Can you work these out from the model? Positions are in its coordinate system, mm. A direction names the side the tool comes from. Round coordinates to 2 decimals unless told otherwise and drop trailing zeros. Loops run counter-clockwise (first coordinate to the right, second up) from the corner with the lowest first, then second, coordinate; pieces in that order, holes last. Notation, with made-up numbers: (74, -9) -> (114, -9) arc R8 cw to (114, 2) -> close; hole circle Ø9 at (84, -33.5). An arc over 180 degrees is marked (long way). Answer as a JSON object with one key per item and string values.
```python
from build123d import *

# Parameters (mm, degrees)
EXTRUDE_THIN4_DEPTH   = 96.52
EXTRUDE_THIN4_2_DEPTH = 96.52
SKETCH5_W             = 32.004
SKETCH5_H             = 76.792210726
CUT_EXTRUDE2_DEPTH    = 26.67
SKETCH6_W             = 32.512
SKETCH6_H             = 76.792210726
CUT_EXTRUDE3_DEPTH    = 26.67
SKETCH7_W             = 152.4
SKETCH7_H             = 25.4
BOSS_EXTRUDE1_DEPTH   = 26.67
BOSS_EXTRUDE2_DEPTH   = 12.7
SKETCH13_W            = 25.4
SKETCH13_H            = 19.05
BOSS_EXTRUDE3_DEPTH   = 12.7


with BuildPart() as part:
    # Sketch1 → Extrude-Thin4 (new body)
    with BuildSketch(Plane(origin=(0, 0, 0), x_dir=(0, 0, -1), z_dir=(1, 0, 0))):
        Polygon((19.05, -1.27), (55.88, -1.27), (55.88, -50.207789274), (-2.03892683, -98.807539415), (-0.406246301, -100.753292301), (58.42, -51.392210726), (58.42, 1.27), (19.05, 1.27), align=None)
    extrude(amount=EXTRUDE_THIN4_DEPTH)

    # Sketch6 → Cut-Extrude3 (cut)
    with BuildSketch(Plane(origin=(0, -58.924421698, -49.443460514), x_dir=(1, 0, 0), z_dir=(0, -0.7660444431189791, -0.6427876096865379))):
        with Locations((48.26, 26.678065285)):
            Rectangle(SKETCH6_W, SKETCH6_H)
    extrude(amount=-CUT_EXTRUDE3_DEPTH, mode=Mode.SUBTRACT)



with BuildPart() as body_2:
    # Sketch1 → Extrude-Thin4 2 (new body)
    with BuildSketch(Plane(origin=(0, 0, 0), x_dir=(0, 0, -1), z_dir=(1, 0, 0))):
        Polygon((-19.05, 1.27), (-58.42, 1.27), (-58.42, -51.392210726), (0.406246301, -100.753292301), (2.03892683, -98.807539415), (-55.88, -50.207789274), (-55.88, -1.27), (-19.05, -1.27), align=None)
    extrude(amount=EXTRUDE_THIN4_2_DEPTH)

    # Sketch5 → Cut-Extrude2 (cut)
    with BuildSketch(Plane(origin=(0, -58.924421698, 49.443460514), x_dir=(1, 0, 0), z_dir=(0, -0.7660444431189799, 0.6427876096865373))):
        with Locations((16.002, -26.678065285)):
            Rectangle(SKETCH5_W, SKETCH5_H)
        with Locations((80.518, -26.678065285)):
            Rectangle(SKETCH5_W, SKETCH5_H)
    extrude(amount=-CUT_EXTRUDE2_DEPTH, mode=Mode.SUBTRACT)


with BuildPart() as part_1:
    add(part.part)

    add(body_2.part)  # Boss-Extrude1 merges body 2
    # Sketch7 → Boss-Extrude1 (add)
    with BuildSketch(Plane(origin=(96.52, 0, 0), x_dir=(0, 0, -1), z_dir=(1, 0, 0))):
        Rectangle(SKETCH7_W, SKETCH7_H)
    extrude(amount=BOSS_EXTRUDE1_DEPTH)

    # Sketch8 → Boss-Extrude2 (add)
    with BuildSketch(Plane.ZY.offset(-96.52)):
        Polygon((0, -12.7), (0, 12.7), (-19.05, 12.7), (-19.05, 1.27), (-19.05, -1.27), (-19.05, -12.7), align=None)
        Polygon((19.05, 1.27), (19.05, 12.7), (0, 12.7), (0, -12.7), (19.05, -12.7), (19.05, -1.27), align=None)
    extrude(amount=BOSS_EXTRUDE2_DEPTH)

    # Sketch13 → Boss-Extrude3 (add)
    with BuildSketch(Plane.ZY.offset(-96.52)):
        with Locations((-58.42, 1.27)):
            Rectangle(SKETCH13_W, SKETCH13_H)
        with Locations((58.42, 1.27)):
            Rectangle(SKETCH13_W, SKETCH13_H)
    extrude(amount=BOSS_EXTRUDE3_DEPTH)


solid = part_1.part
```
Q1. I want a section at C-C, the plane z = 22.5. Write out the boundary of the cut face in (x, y).
Determined:
{"outline": "(0, -1.27) -> (96.52, -1.27) -> (96.52, -12.7) -> (123.19, -12.7) -> (123.19, 12.7) -> (96.52, 12.7) -> (96.52, 1.27) -> (0, 1.27) -> close; (32, -81.53) -> (64.52, -81.53) -> (64.52, -78.22) -> (32, -78.22) -> close"}
Q2. I'm going to push flat-ended pins straight in: pin 1 (5.5 mm diameter, centred on x = 92, y = -6, fed in from -Z); pin 2 (2 mm diameter, centred on x = 58, z = 34, fed in from +Y); pin 3 (10 mm diameter, centred on x = 104, y = -71, fed in from +Z); pin 4 (1 mm diameter, centred on x = 32, z = 12, fed in from -Y). Where does each tip first touch, or does it pass through?
Determined:
{"pin 1": "z = -71.12", "pin 2": "y = 1.27", "pin 3": "through", "pin 4": "y = -90.76"}
Q3. I want a section at A-A, the plane y = -20. Write out the boundary of the cut face in (x, z).
Determined:
{"outline": "(0, -58.42) -> (96.52, -58.42) -> (96.52, -55.88) -> (0, -55.88) -> close; (0, 55.88) -> (96.52, 55.88) -> (96.52, 58.42) -> (0, 58.42) -> close"}
Q4. We'd pull the mould along Z, two halves only. Please class faces 5 (the flat face through (123.19, 0, 1)), 6 (the flat face through (90, 6, -45.72)), 7 (the flat face through (90, -7, 19.05)), 8 (the flat face through (48.032, -75.727, 29.419)): pulls with the +Z half, pulls with the -Z half, needs draft (parallel to the pull), parting line crosses it, or undercut.
Determined:
{"face 5": "needs draft", "face 6": "undercut", "face 7": "undercut", "face 8": "pulls with the +Z half"}
Q5. On a 3-axis mill with a long thin cutter (end or side, diameter ignored), from which of +Z, -Z, +X, -X, +Y, -Y can I reach the whole of each face in a straight line? I mean faces 1 (the flat face through (90, 1, 71.12)), 2 (the flat face through (83.82, -5, -51)), 3 (the flat face through (90, -8.255, 51)), 4 (the flat face through (90, 7, 19.05)). Say none if no direction works.
Determined:
{"face 1": "+Z, -X, +Y, -Y", "face 2": "-X", "face 3": "-X, -Y", "face 4": "-X, +Y"}
Q6. If I drill on L1, parallel to Z at x = 22.5, y = -30; L2, parallel to Z at x = 49, y = 1; L3, parallel to Y at x = 91, z = 26, over which ranges is the centre line in solid material (lowest first)? Write a range as [from, to].
Determined:
{"L1": "[-58.42, -55.88], [55.88, 58.42]", "L2": "[-58.42, -19.05], [19.05, 58.42]", "L3": "[-1.27, 1.27]"}
Q7. I want a section at B-B, the plane x = 36.5. Write out the boundary of the cut face in (y, z).
Determined:
{"outline": "(-100.75, -0.41) -> (-98.81, -2.04) -> (-50.21, 55.88) -> (-1.27, 55.88) -> (-1.27, 19.05) -> (1.27, 19.05) -> (1.27, 58.42) -> (-51.39, 58.42) -> close; (-51.39, -58.42) -> (1.27, -58.42) -> (1.27, -19.05) -> (-1.27, -19.05) -> (-1.27, -55.88) -> (-48.37, -55.88) -> close"}
Q8. I want a section at D-D, the plane y = -83.5. Write out the boundary of the cut face in (x, z).
Determined:
{"outline": "(0, -20.16) -> (32, -20.16) -> (32, -16.2) -> (0, -16.2) -> close; (32, 16.2) -> (64.52, 16.2) -> (64.52, 20.16) -> (32, 20.16) -> close; (64.52, -20.16) -> (96.52, -20.16) -> (96.52, -16.2) -> (64.52, -16.2) -> close"}
